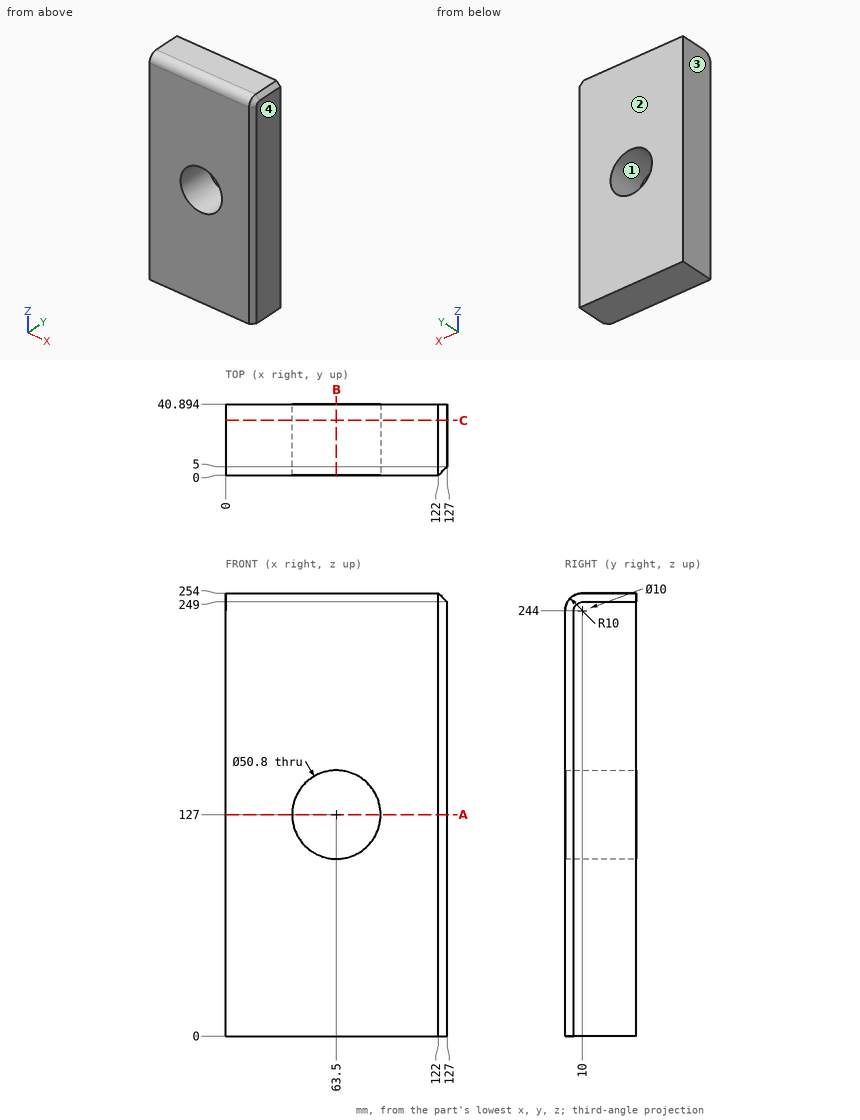
Study the drawing (mm; zero at the part's minimum x, y, z) and answer. Coordinates: 2 decimals unless noted, no trailing zeros. Order: outer loops, then holes, each group sorted by start corner. A loop starts at its lowest first (then second) coordinate and runs counter-clockwise, first axis right, second up. Notation, with made-up numbers: M 8,39.25 L 32,39.25 A32 ccw 32,71.25 Z; hole C 67.5,-34 d1. An arc over 180 degrees is marked long. Answer as a JSON object with one key per item and string values. Group by question number.
1. Straight lines are drawn through the part: line 1 (Z direction, x = 63, y = 25); line 2 (Z direction, x = 66, y = 37); line 3 (Z direction, x = 116, y = 8). For each, find the intervals that lie inside material, in ascending order.
2. Section C-C on y = 31.5 is taken. Write down the section's boundary in (x, z).
3. Section A-A on z = 127 is taken. Write down the section's boundary in (x, y).
4. Determine the mould class of the marked faces 1, 2, 3 and 4 for opening direction X: released by +X, released by -X, zero draft, split by the parting line, or undercut.
5. Section B-B on x = 63.5 is taken. Write down the section's boundary in (y, z).
Values follow:
{
 "1": {"line 1": "0 to 101.6, 152.4 to 254", "line 2": "0 to 101.72, 152.28 to 254", "line 3": "0 to 253.8"},
 "2": {"outline": "M 0,0 L 127,0 L 127,249 L 122,254 L 0,254 Z; hole C 63.5,127 d50.8"},
 "3": {"outline": "M 0,0 L 38.1,0 L 38.1,40.89 L 0,40.89 Z; M 88.9,0 L 122,0 L 127,5 L 127,40.89 L 88.9,40.89 Z"},
 "4": {"face 1": "undercut", "face 2": "zero draft", "face 3": "released by -X", "face 4": "released by +X"},
 "5": {"outline": "M 0,0 L 40.89,0 L 40.89,101.6 L 0,101.6 Z; M 0,152.4 L 40.89,152.4 L 40.89,254 L 10,254 A10 ccw 0,244 Z"}
}
